Build history of the part. All positions in model axes, mm. Give positions to 0.01 mm unless a question says otherwise; leave off trailing zeros. Write each loop counter-clockwise with the first axis right and the second up, starting at its lowest first coordinate (ties: lowest second). Pieces come first, ordered by that corner, then holes. Notation, with made-up numbers: (81.25, 42.5) -> (92.25, 42.5) arc R9 cw to (92.25, 58.5) -> close; hole circle Ø9 at (19, 20). An arc over 180 degrees is marked (long way). Put each result on its own line as item: value. Start each with the question number.
Item 1: Slice it at C-C, the plane x = -64. List the corners of the cut face in (y, z).
Item 2: Flat gauge pins, fed straight in: pin 1 Ø6.5 at (x, z) = (20.25, 20.25) entering from +Y; pin 2 Ø1 at (x, y) = (35.5, 0.5) entering from +Z. Where does each tip first touch, or does it go through?
Item 3: Drill centre lines: line 1 along X through (y, z) = (-0.65, -56.5); line 2 along X through (y, z) = (0.2, 53.5); line 3 along Z through (x, y) = (-24, 0.6). Where is each one in solid material? Low to high.
Item 4: Slice it at B-B, the plane z = -51. List the corners of the cut face in (x, y), plus the area to 3 significant figures.
Item 5: Slice it at A-A, the plane y = -0.6. List the corners of the cut face in (x, z).
```python
from build123d import *

# Parameters (mm, degrees)
BOSS_EXTRUDE1_DEPTH      = 1.5
BOSS_EXTRUDE1_DEPTH_BACK = 1.5
SKETCH1_R                = 73.2
SKETCH1_R_2              = 2


with BuildPart() as part:
    # Sketch1 → Boss-Extrude1 (new, two sides: drawn at the far end of the back side and taken through both)
    with BuildSketch(Plane(origin=(0, 0, 0), x_dir=(1, 0, 0), z_dir=(0, 1, 0)).offset(-BOSS_EXTRUDE1_DEPTH_BACK)):
        with Locations(Location((0, 0, 0), (0, 0, 270))):
            Circle(SKETCH1_R)
        with Locations(Location((20.253785579, 20.253785579, 0), (0, 0, 270))):
            Circle(SKETCH1_R_2, mode=Mode.SUBTRACT)
        with Locations(Location((20.253785579, -20.253785579, 0), (0, 0, 270))):
            Circle(SKETCH1_R_2, mode=Mode.SUBTRACT)
        with Locations(Location((-20.253785579, -20.253785579, 0), (0, 0, 270))):
            Circle(SKETCH1_R_2, mode=Mode.SUBTRACT)
        with Locations(Location((-20.253785579, 20.253785579, 0), (0, 0, 270))):
            Circle(SKETCH1_R_2, mode=Mode.SUBTRACT)
    extrude(amount=BOSS_EXTRUDE1_DEPTH + BOSS_EXTRUDE1_DEPTH_BACK)


solid = part.part
```
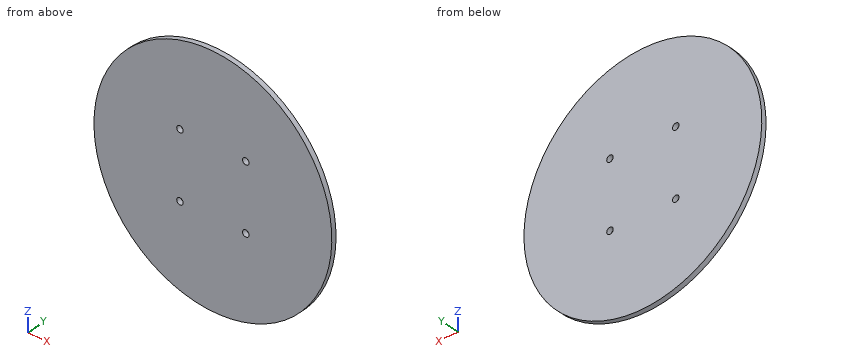
Values follow:
1. outline: (-1.5, -35.53) -> (1.5, -35.53) -> (1.5, 35.53) -> (-1.5, 35.53) -> close
2. pin 1: y = 1.5
2. pin 2: z = 64.29
3. line 1: -46.54 to 46.54
3. line 2: -49.96 to 49.96
3. line 3: -69.15 to 69.15
4. outline: (-52.51, -1.5) -> (52.51, -1.5) -> (52.51, 1.5) -> (-52.51, 1.5) -> close
4. area: 315 mm2
5. outline: circle Ø146.4 at (0, 0); hole circle Ø4 at (-20.25, -20.25); hole circle Ø4 at (-20.25, 20.25); hole circle Ø4 at (20.25, -20.25); hole circle Ø4 at (20.25, 20.25)
